Here's the drawing with two shaded views (mm, measured from the low corner). I have some questions. Give positions to 0.01 mm unless a question says otherwise; leave off trailing zeros. Write each loop counter-clockwise with the first axis right and the second up, starting at its lowest first coordinate (ties: lowest second). Pieces come first, ordered by that corner, then holes. Notation, with made-up numbers: (6.25, 35.25) -> (26.25, 35.25) arc R34 cw to (26.25, 65.25) -> close; hole circle Ø9 at (47.5, 11.25). An arc over 180 degrees is marked (long way). One line per item, written item: value.
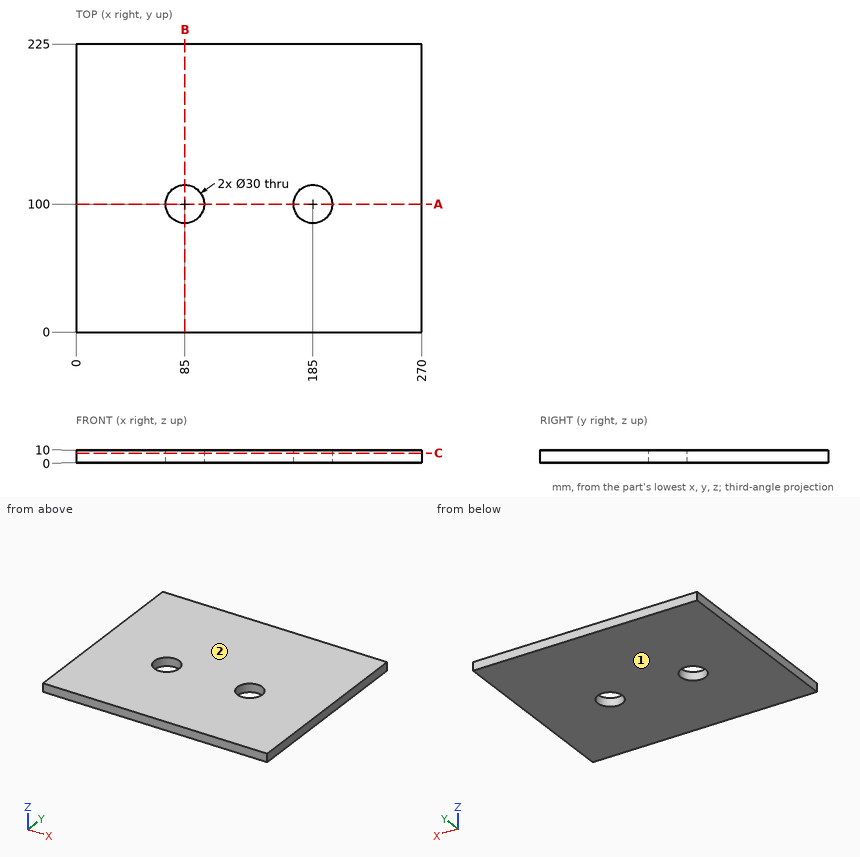
1) If we section it at A-A (y = 100): Write out the boundary of the cut face in (x, z).
Answer list:
outline: (0, 0) -> (70, 0) -> (70, 10) -> (0, 10) -> close; (100, 0) -> (170, 0) -> (170, 10) -> (100, 10) -> close; (200, 0) -> (270, 0) -> (270, 10) -> (200, 10) -> close
2) Will this pin go through, and if not, where does the flat tip stop? pin 1 (24 mm diameter, centred on x = 185, y = 100, fed in from +Z).
Answer list:
pin 1: passes through
3) If we section it at B-B (x = 85): Write out the boundary of the cut face in (y, z).
Answer list:
outline: (0, 0) -> (85, 0) -> (85, 10) -> (0, 10) -> close; (115, 0) -> (225, 0) -> (225, 10) -> (115, 10) -> close
4) If we section it at C-C (z = 7.75): Write out the boundary of the cut face in (x, y).
Answer list:
outline: (0, 0) -> (270, 0) -> (270, 225) -> (0, 225) -> close; hole circle Ø30 at (85, 100); hole circle Ø30 at (185, 100)
5) I need wall thicknesses on L1, parallel to X at y = 100, z = 6.75; L2, parallel to Y at x = 185, z = 5.75; L3, parallel to Y at x = 75, z = 7.75. Which ranges of each line are inside material? Lowest first, please.
Answer list:
L1: x = 0 to 70, 100 to 170, 200 to 270
L2: y = 0 to 85, 115 to 225
L3: y = 0 to 88.82, 111.18 to 225
6) We'd pull the mould along Z, two halves only. Please class the marked faces 1 and 2: released by +Z, released by -Z, zero draft, split by the parting line, or undercut.
Answer list:
face 1: released by -Z
face 2: released by +Z
